```python
from build123d import *

# Parameters (mm, degrees)
F0_W     = 60
F0_H     = 70
F1_DEPTH = 15
F2_DEPTH = 50
F3_DEPTH = 53
F4_DEPTH = 3


with BuildPart() as f1:
    # F0 (on Top) → F1 (new body)
    with BuildSketch(Plane.XY):
        Rectangle(F0_W, F0_H)
        with BuildLine():
            Line((0, 21), (14.5, 21))
            ThreePointArc((14.5, 21), (19.5, 26), (24.5, 21))
            ThreePointArc((24.5, 21), (23.0355339059, 17.4644660941), (19.5, 16))
            Line((19.5, 16), (19.5, 0))
            Line((19.5, 0), (19.5, -16))
            ThreePointArc((19.5, -16), (23.0355339059, -17.4644660941), (24.5, -21))
            ThreePointArc((24.5, -21), (19.5, -26), (14.5, -21))
            Line((14.5, -21), (0, -21))
            Line((0, -21), (-14.5, -21))
            ThreePointArc((-14.5, -21), (-23.0355339059, -24.5355339059), (-19.5, -16))
            Line((-19.5, -16), (-19.5, 16))
            ThreePointArc((-19.5, 16), (-23.0355339059, 24.5355339059), (-14.5, 21))
            Line((-14.5, 21), (0, 21))
        make_face(mode=Mode.SUBTRACT)
        with BuildLine():
            ThreePointArc((19.5, 16), (15.9644660941, 17.4644660941), (14.5, 21))
            Line((14.5, 21), (0, 21))
            ThreePointArc((0, 21), (4.2426406871, 19.2426406871), (6, 15))
            ThreePointArc((6, 15), (4.2426406871, 10.7573593129), (0, 9))
            Line((0, 9), (0, 0))
            Line((0, 0), (19.5, 0))
            Line((19.5, 0), (19.5, 16))
        make_face()
        with BuildLine():
            ThreePointArc((0, 9), (-6, 15), (0, 21))
            Line((0, 21), (-14.5, 21))
            ThreePointArc((-14.5, 21), (-15.9644660941, 17.4644660941), (-19.5, 16))
            Line((-19.5, 16), (-19.5, -16))
            ThreePointArc((-19.5, -16), (-15.9644660941, -17.4644660941), (-14.5, -21))
            Line((-14.5, -21), (0, -21))
            ThreePointArc((0, -21), (-6, -15), (0, -9))
            Line((0, -9), (0, 0))
            Line((0, 0), (0, 9))
        make_face()
        with BuildLine():
            Line((19.5, -16), (19.5, 0))
            Line((19.5, 0), (0, 0))
            Line((0, 0), (0, -9))
            ThreePointArc((0, -9), (4.2426406871, -10.7573593129), (6, -15))
            ThreePointArc((6, -15), (4.2426406871, -19.2426406871), (0, -21))
            Line((0, -21), (14.5, -21))
            ThreePointArc((14.5, -21), (15.9644660941, -17.4644660941), (19.5, -16))
        make_face()
    extrude(amount=F1_DEPTH)

    # F0 (on Top) → F2 (join)
    with BuildSketch(Plane.XY):
        with BuildLine():
            ThreePointArc((19.5, 19), (18.0857864376, 19.5857864376), (17.5, 21))
            Line((17.5, 21), (14.5, 21))
            ThreePointArc((14.5, 21), (15.9644660941, 17.4644660941), (19.5, 16))
            Line((19.5, 16), (19.5, 19))
        make_face()
        with BuildLine():
            ThreePointArc((17.5, 21), (19.5, 23), (21.5, 21))
            ThreePointArc((21.5, 21), (20.9142135624, 19.5857864376), (19.5, 19))
            Line((19.5, 19), (19.5, 16))
            ThreePointArc((19.5, 16), (23.0355339059, 17.4644660941), (24.5, 21))
            ThreePointArc((24.5, 21), (19.5, 26), (14.5, 21))
            Line((14.5, 21), (17.5, 21))
        make_face()
        with BuildLine():
            Line((-17.5, 21), (-14.5, 21))
            ThreePointArc((-14.5, 21), (-23.0355339059, 24.5355339059), (-19.5, 16))
            Line((-19.5, 16), (-19.5, 19))
            ThreePointArc((-19.5, 19), (-20.9142135624, 22.4142135624), (-17.5, 21))
        make_face()
        with BuildLine():
            ThreePointArc((-19.5, 16), (-15.9644660941, 17.4644660941), (-14.5, 21))
            Line((-14.5, 21), (-17.5, 21))
            ThreePointArc((-17.5, 21), (-18.0857864376, 19.5857864376), (-19.5, 19))
            Line((-19.5, 19), (-19.5, 16))
        make_face()
        with BuildLine():
            ThreePointArc((-14.5, -21), (-15.9644660941, -17.4644660941), (-19.5, -16))
            Line((-19.5, -16), (-19.5, -19))
            ThreePointArc((-19.5, -19), (-18.0857864376, -19.5857864376), (-17.5, -21))
            Line((-17.5, -21), (-14.5, -21))
        make_face()
        with BuildLine():
            Line((-19.5, -19), (-19.5, -16))
            ThreePointArc((-19.5, -16), (-23.0355339059, -24.5355339059), (-14.5, -21))
            Line((-14.5, -21), (-17.5, -21))
            ThreePointArc((-17.5, -21), (-20.9142135624, -22.4142135624), (-19.5, -19))
        make_face()
        with BuildLine():
            Line((19.5, -19), (19.5, -16))
            ThreePointArc((19.5, -16), (15.9644660941, -17.4644660941), (14.5, -21))
            Line((14.5, -21), (17.5, -21))
            ThreePointArc((17.5, -21), (18.0857864376, -19.5857864376), (19.5, -19))
        make_face()
        with BuildLine():
            ThreePointArc((24.5, -21), (23.0355339059, -17.4644660941), (19.5, -16))
            Line((19.5, -16), (19.5, -19))
            ThreePointArc((19.5, -19), (20.9142135624, -19.5857864376), (21.5, -21))
            ThreePointArc((21.5, -21), (19.5, -23), (17.5, -21))
            Line((17.5, -21), (14.5, -21))
            ThreePointArc((14.5, -21), (19.5, -26), (24.5, -21))
        make_face()
    extrude(amount=F2_DEPTH)

    # F0 (on Top) → F3 (join)
    with BuildSketch(Plane.XY):
        with BuildLine():
            ThreePointArc((-17.5, -21), (-18.0857864376, -19.5857864376), (-19.5, -19))
            Line((-19.5, -19), (-19.5, -21))
            Line((-19.5, -21), (-17.5, -21))
        make_face()
        with BuildLine():
            Line((-19.5, -21), (-19.5, -19))
            ThreePointArc((-19.5, -19), (-20.9142135624, -22.4142135624), (-17.5, -21))
            Line((-17.5, -21), (-19.5, -21))
        make_face()
        with BuildLine():
            Line((-19.5, 21), (-17.5, 21))
            ThreePointArc((-17.5, 21), (-20.9142135624, 22.4142135624), (-19.5, 19))
            Line((-19.5, 19), (-19.5, 21))
        make_face()
        with BuildLine():
            ThreePointArc((-19.5, 19), (-18.0857864376, 19.5857864376), (-17.5, 21))
            Line((-17.5, 21), (-19.5, 21))
            Line((-19.5, 21), (-19.5, 19))
        make_face()
        with BuildLine():
            Line((19.5, -21), (19.5, -19))
            ThreePointArc((19.5, -19), (18.0857864376, -19.5857864376), (17.5, -21))
            Line((17.5, -21), (19.5, -21))
        make_face()
        with BuildLine():
            ThreePointArc((21.5, -21), (20.9142135624, -19.5857864376), (19.5, -19))
            Line((19.5, -19), (19.5, -21))
            Line((19.5, -21), (17.5, -21))
            ThreePointArc((17.5, -21), (19.5, -23), (21.5, -21))
        make_face()
        with BuildLine():
            Line((19.5, 21), (17.5, 21))
            ThreePointArc((17.5, 21), (18.0857864376, 19.5857864376), (19.5, 19))
            Line((19.5, 19), (19.5, 21))
        make_face()
        with BuildLine():
            ThreePointArc((19.5, 19), (20.9142135624, 19.5857864376), (21.5, 21))
            ThreePointArc((21.5, 21), (19.5, 23), (17.5, 21))
            Line((17.5, 21), (19.5, 21))
            Line((19.5, 21), (19.5, 19))
        make_face()
    extrude(amount=F3_DEPTH)

    # F0 (on Top) → F4 (join)
    with BuildSketch(Plane.XY):
        with BuildLine():
            ThreePointArc((6, 15), (4.2426406871, 19.2426406871), (0, 21))
            ThreePointArc((0, 21), (-6, 15), (0, 9))
            ThreePointArc((0, 9), (4.2426406871, 10.7573593129), (6, 15))
        make_face()
        with BuildLine():
            ThreePointArc((2, 15), (1.4142135624, 13.5857864376), (0, 13))
            ThreePointArc((0, 13), (-1.4142135624, 16.4142135624), (2, 15))
        make_face(mode=Mode.SUBTRACT)
        with BuildLine():
            ThreePointArc((6, -15), (4.2426406871, -10.7573593129), (0, -9))
            ThreePointArc((0, -9), (-6, -15), (0, -21))
            ThreePointArc((0, -21), (4.2426406871, -19.2426406871), (6, -15))
        make_face()
        with BuildLine():
            ThreePointArc((2, -15), (-1.4142135624, -16.4142135624), (0, -13))
            ThreePointArc((0, -13), (1.4142135624, -13.5857864376), (2, -15))
        make_face(mode=Mode.SUBTRACT)
    extrude(amount=F4_DEPTH)


solid = f1.part
```
Part model, mm, in its own coordinate system. A direction names the side the tool comes from. Round coordinates to 2 decimals unless told otherwise and drop trailing zeros. Loops run counter-clockwise (first coordinate to the right, second up) from the corner with the lowest first, then second, coordinate; pieces in that order, holes last. Notation, with made-up numbers: (-9.5, 58) -> (33.5, 58) arc R20 ccw to (33.5, 69) -> close; hole circle Ø3 at (25, 5). An arc over 180 degrees is marked (long way). Use a Markdown table: item, result.
1) Cut at B-B, the plane z = 7. List the corners of the cut face in (x, y).
The answers:
| item | result |
|---|---|
| outline | (-30, -35) -> (30, -35) -> (30, 35) -> (-30, 35) -> close; hole circle Ø12 at (0, -15); hole circle Ø12 at (0, 15) |
2) Probe line 1 (X direction, y = 15, z = 1); line 2 (Z direction, x = -14, y = 15); line 3 (Y direction, x = -19.5, z = 18). List the from-to ranges inside material, lowest first. Write a range as [from, to].
The answers:
| item | result |
|---|---|
| line 1 | x = [-30, -2], [2, 30] |
| line 2 | z = [0, 15] |
| line 3 | y = [-26, -16], [16, 26] |
3) Tool access for faces 1 (the flat face through (-20, -21, 53)), 2 (the flat face through (0, -18, 3)): list every direction of +Z, -Z, +X, -X, +Y, -Y with a clear straight run to the whole face (end or side of a thin tool).
The answers:
| item | result |
|---|---|
| face 1 | +Z, +X, -X, +Y, -Y |
| face 2 | +Z |
4) Drop flat-ended pins along their axis: pin 1 Ø1.5 at (y, z) = (22, 19) entering from -X; pin 2 Ø13 at (x, y) = (0.5, -14) entering from +Z; pin 3 Ø3.5 at (x, y) = (-2, 17.5) entering from +Z. Give the stop position or say it passes through.
The answers:
| item | result |
|---|---|
| pin 1 | stops at x = -24.49 |
| pin 2 | stops at z = 15 |
| pin 3 | stops at z = 3 |
5) Cut at C-C, the plane x = 16. List the corners of the cut face in (y, z), and give its area (3 significant figures).
The answers:
| item | result |
|---|---|
| outline | (-35, 0) -> (35, 0) -> (35, 15) -> (24.57, 15) -> (24.57, 50) -> (17.43, 50) -> (17.43, 15) -> (-17.43, 15) -> (-17.43, 50) -> (-24.57, 50) -> (-24.57, 15) -> (-35, 15) -> close |
| area | 1,550 mm2 |
6) Pull direction X, two halves, no side cores. Call faces 3 (the flat face through (30, 0, 7)), 4 (the flat face through (0, 12, 3)), 5 (the flat face through (-20, 21, 53)), 6 (the flat face through (-30, 0, 7)): pulls with the +X half, pulls with the -X half, needs draft (parallel to the pull), parting line crosses it, or undercut.
The answers:
| item | result |
|---|---|
| face 3 | pulls with the +X half |
| face 4 | undercut |
| face 5 | needs draft |
| face 6 | pulls with the -X half |
7) Cut at D-D, the plane y = 3.5. List the corners of the cut face in (x, z), and give its area (3 significant figures).
The answers:
| item | result |
|---|---|
| outline | (-30, 0) -> (30, 0) -> (30, 15) -> (-30, 15) -> close |
| area | 900 mm2 |
8) Cut at A-A, the plane z = 49. List the corners of the cut face in (x, y).
The answers:
| item | result |
|---|---|
| outline | circle Ø10 at (-19.5, -21); circle Ø10 at (-19.5, 21); circle Ø10 at (19.5, -21); circle Ø10 at (19.5, 21) |
